Read the model definition and answer for the solid it produces. Units are mm, in the model's axes. Face numbers are marked on the shaded views. Give positions to 0.01 mm unless a question says otherwise; leave off trailing zeros. Order: outer loops, then holes, each group sorted by start corner. A loop starts at its lowest first (then second) coordinate and runs counter-clockwise, first axis right, second up. Notation, with made-up numbers: (-21, 70) -> (21, 70) arc R14 cw to (21, 82) -> close; hole circle Ø3 at (76.25, 0). An arc over 180 degrees is marked (long way). One line per item, written item: value. Start each with the question number.
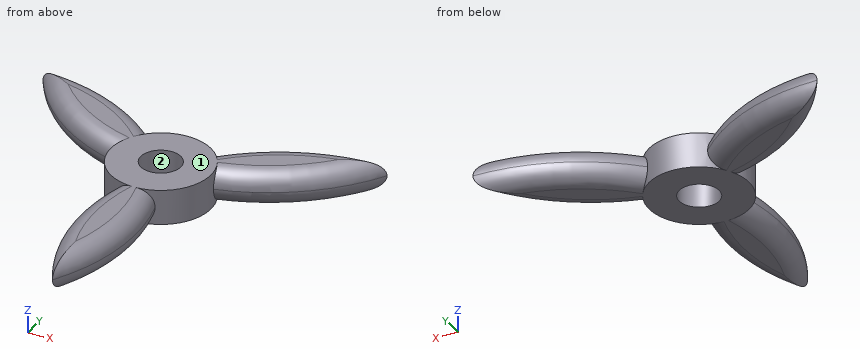
from build123d import *

# Parameters (mm, degrees)
SKETCH1_R           = 4
BOSS_EXTRUDE1_DEPTH = 7
FILLET2_R           = 3.5


with BuildPart() as part:
    # Sketch1 → Boss-Extrude1 (new body)
    with BuildSketch(Plane.XY):
        with BuildLine():
            ThreePointArc((-9.921567416, 1.25), (-8.660254038, -5), (-3.878251954, -9.217329428))
            ThreePointArc((-3.878251954, -9.217329428), (-5.045253515, -25), (0, -40))
            ThreePointArc((0, -40), (5.045253515, -25), (3.878251954, -9.217329428))
            ThreePointArc((3.878251954, -9.217329428), (8.660254038, -5), (9.921567416, 1.25))
            ThreePointArc((9.921567416, 1.25), (24.173261852, 8.130682288), (34.641016151, 20))
            ThreePointArc((34.641016151, 20), (19.128008337, 16.869317712), (6.043315463, 7.967329428))
            ThreePointArc((6.043315463, 7.967329428), (0, 10), (-6.043315463, 7.967329428))
            ThreePointArc((-6.043315463, 7.967329428), (-19.128008337, 16.869317712), (-34.641016151, 20))
            ThreePointArc((-34.641016151, 20), (-24.173261852, 8.130682288), (-9.921567416, 1.25))
        make_face()
        Circle(SKETCH1_R, mode=Mode.SUBTRACT)
    extrude(amount=BOSS_EXTRUDE1_DEPTH)

    # Fillet2
    fillet2_edges = [part.edges().sort_by_distance(p)[0] for p in [
        (-19.128008337, 16.869317712, 0),
        (-24.173261852, 8.130682288, 0),
        (19.128008337, 16.869317712, 0),
        (24.173261852, 8.130682288, 0),
        (5.045253515, -25, 0),
        (-5.045253515, -25, 0),
        (-5.045253515, -25, 7),
        (5.045253515, -25, 7),
        (24.173261852, 8.130682288, 7),
        (19.128008337, 16.869317712, 7),
        (-19.128008337, 16.869317712, 7),
        (-24.173261852, 8.130682288, 7),
    ]]
    fillet(fillet2_edges, radius=FILLET2_R - 0.0001)  # a hair under: the kernel refuses the full size


solid = part.part
Item 1: For a pull along Y with two mould halves and no side action, classify the marked faces 1 and 2 as +Y half, -Y half, draft (parallel to the pull), parting line (faces both ways), or undercut.
Item 2: Find the intervals of material crossed by line 1 (X direction, y = -1.5, z = 1.75); line 2 (X direction, y = -3, z = 4.75); line 3 (Z direction, x = 14, y = 6), in increasing order. Write a range as from..to.
Item 3: Flat-ended cylindrical pins translate along their axes: pin 1 (4 mm diameter, centred on x = -19.5, z = 6, fed in from +Y); pin 2 (1.5 mm diameter, centred on y = 12.5, z = 4.5, fed in from +X); pin 3 (2 mm diameter, centred on x = -11.5, y = 6, fed in from -Z); pin 4 (4 mm diameter, centred on y = 6, z = 4.5, fed in from -X). Find the tip coordinate at first contact, or state that the pin passes through.
Item 4: Find section A-A on y = 0. Write down the section's boundary in (x, z).
Item 5: Find section B-B on z = 5.5. Write down the section's boundary in (x, y).
Checks:
1. face 1: draft
1. face 2: undercut
2. line 1: -9.89..-3.71, 3.71..9.89
2. line 2: -9.54..-2.65, 2.65..9.54
2. line 3: 0.01..6.99
3. pin 1: y = 17.39
3. pin 2: x = 29.59
3. pin 3: z = 0
3. pin 4: x = -23.86
4. outline: (-10, 0) -> (-4, 0) -> (-4, 7) -> (-10, 7) -> close; (4, 0) -> (10, 0) -> (10, 7) -> (4, 7) -> close
5. outline: (-33.53, 19.36) arc R39.37 ccw to (-9.82, 1.87) arc R10 ccw to (-3.29, -9.44) arc R39.37 ccw to (0, -38.71) arc R39.37 ccw to (3.29, -9.44) arc R10 ccw to (9.82, 1.87) arc R39.37 ccw to (33.53, 19.36) arc R39.37 ccw to (6.53, 7.57) arc R10 ccw to (-6.53, 7.57) arc R39.37 ccw to start; hole circle Ø8 at (0, 0)
